Work out the finished part from the listing and answer in its coordinate system (mm). A direction names the side the tool comes from. Round coordinates to 2 decimals unless told otherwise and drop trailing zeros. Order: outer loops, then holes, each group sorted by start corner. A loop starts at its lowest first (then second) coordinate and runs counter-clockwise, first axis right, second up. Notation, with made-up numbers: (-25.5, 20.25) - (-9.5, 20.25) arc R19 cw to (-9.5, 41.25) - close; hole circle Ø10 at (-12.5, 61). An arc over 180 degrees is marked (long way). One line per question, with ' | ' between items. Start each with the question number.
Solid Edge part; units mm, degrees
sketch "Sketch1" plane through (0, 0, 0) normal (0, 0, 1) x (1, 0, 0)
  line L0 (-60, 45) -> (-60, -45)
  line L1 (-60, -45) -> (60, -45)
  line L2 (60, -45) -> (60, 45)
  line L3 (60, 45) -> (-60, 45)
extrude "Protrusion1" add sketch "Sketch1" along normal blind 15
sketch "Sketch2" plane through (0, 0, 15) normal (0, 0, 1) x (1, 0, 0)
  circle A0 centre (0, 0) radius 20
extrude "Cutout1" cut sketch "Sketch2" against normal through all
sketch "Sketch3" plane through (0, 0, 15) normal (0, 0, 1) x (1, 0, 0)
  line L0 (-60, -7.5) -> (110, -7.5)
  line L1 (110, -7.5) -> (110, 7.5)
  line L2 (110, 7.5) -> (-60, 7.5)
  line L3 (-60, 7.5) -> (-60, -7.5)
  dimension "D1" = 60
  dimension "D2" = 60
extrude "VaciadoExtruido_2" cut sketch "Sketch3" against normal blind 5
chamfer "Chaflán_1" distance 5 angle 45 4 edges at (-60, 45, 7.5) (60, 45, 7.5) (60, -45, 7.5) (-60, -45, 7.5)
hole "Agujero_1" [suppressed]
hole "Hole1" at (-35, 0, 0) direction (0, 0, 1) diameter 7 end up to next counterbore diameter 11 counterbore depth 6.8
hole "Hole2" at (50, 0, 0) direction (0, 0, 1) diameter 7 end up to next counterbore diameter 11 counterbore depth 6.8
hole "Agujero_4" at (-43, 38, 15) direction (0, 0, -1) diameter 7 end up to next counterbore diameter 11 counterbore depth 6.8
hole "Hole3" at (43, 38, 15) direction (0, 0, -1) diameter 7 end up to next counterbore diameter 11 counterbore depth 6.8
hole "Hole4" at (43, -38, 15) direction (0, 0, -1) diameter 7 end up to next counterbore diameter 11 counterbore depth 6.8
hole "Hole5" at (-43, -38, 15) direction (0, 0, -1) diameter 7 end up to next counterbore diameter 11 counterbore depth 6.8
hole "Agujero_8" at (0, 38, 15) direction (0, 0, -1) diameter 8 end up to next
hole "Hole6" at (0, -38, 15) direction (0, 0, -1) diameter 8 end up to next
properties part number "1976-1200-002" material "Aluminio, 7075-T6"
1) Section C-C on x = 43 is taken. Give the vertices of the cut face in (y, z), and give its area (3 significant figures).
2) A flat-ended cylindrical pin translates along its axis: pin 1 (5.5 mm diameter, centred on x = 42.5, y = 36, fed in from +Z). Find the tip coordinate at first contact, or state that the pin passes through.
3) For faces 1 (the flat face through (-43, -42, 8.2)), 2 (the cylindrical face through (44.547, -0.716, 3.448)), 3 (the flat face through (-1, 27, 15)), 4 (the flat face through (-40, -7.5, 13)), 5 (the cylindrical face through (46.47, 38.46, 4.16)), determine the directions among +Z, -Z, +X, -X, +Y, -Y from which every point of the face is accessible in a straight line to the end or side of a thin tool.
4) Section D-D on y = 38 is taken. Give the vertices of the cut face in (x, z).
5) Determine the mould class of faces 6 (the flat face through (58, -42, 8)), 7 (the flat face through (-60, 1, 7)), 8 (the cylindrical face through (46.47, -37.54, 4.16)) for opening direction X: released by +X, released by -X, zero draft, split by the parting line, or undercut.
6) Straight lines are drawn through the part: line 1 (X direction, y = 38, z = 12.5); line 2 (Y direction, x = -43, z = 4.75); line 3 (X direction, y = -38, z = 2.25). For each, find the intervals that lie inside material, in ascending order.
7) Section A-A on z = 11.75 is taken. Give the vertices of the cut face in (x, y).
8) Section B-B on y = -12 is taken. Give the vertices of the cut face in (x, z), and give its area (3 significant figures).
Recorded:
1) outline: (-45, 0) - (-41.5, 0) - (-41.5, 8.2) - (-43.5, 8.2) - (-43.5, 15) - (-45, 15) - close; (-34.5, 0) - (34.5, 0) - (34.5, 8.2) - (32.5, 8.2) - (32.5, 15) - (7.5, 15) - (7.5, 10) - (-7.5, 10) - (-7.5, 15) - (-32.5, 15) - (-32.5, 8.2) - (-34.5, 8.2) - close; (41.5, 0) - (45, 0) - (45, 15) - (43.5, 15) - (43.5, 8.2) - (41.5, 8.2) - close | area: 1,010 mm²
2) pin 1: stops at z = 8.2
3) face 1: +Z | face 2: -Z | face 3: +Z, +X, -X, +Y, -Y | face 4: +Z, +X, -X | face 5: +Z, -Z
4) outline: (-60, 0) - (-46.5, 0) - (-46.5, 8.2) - (-48.5, 8.2) - (-48.5, 15) - (-60, 15) - close; (-39.5, 0) - (-4, 0) - (-4, 15) - (-37.5, 15) - (-37.5, 8.2) - (-39.5, 8.2) - close; (4, 0) - (39.5, 0) - (39.5, 8.2) - (37.5, 8.2) - (37.5, 15) - (4, 15) - close; (46.5, 0) - (60, 0) - (60, 15) - (48.5, 15) - (48.5, 8.2) - (46.5, 8.2) - close
5) face 6: released by +X | face 7: released by -X | face 8: undercut
6) line 1: x = -60 to -48.5, -37.5 to -4, 4 to 37.5, 48.5 to 60 | line 2: y = -45 to -41.5, -34.5 to 34.5, 41.5 to 45 | line 3: x = -60 to -46.5, -39.5 to -4, 4 to 39.5, 46.5 to 60
7) outline: (-60, -40) - (-55, -45) - (55, -45) - (60, -40) - (60, -7.5) - (18.54, -7.5) arc R20 cw to (-18.54, -7.5) - (-60, -7.5) - close; (-60, 7.5) - (-18.54, 7.5) arc R20 cw to (18.54, 7.5) - (60, 7.5) - (60, 40) - (55, 45) - (-55, 45) - (-60, 40) - close; hole circle Ø11 at (-43, -38); hole circle Ø11 at (-43, 38); hole circle Ø8 at (0, -38); hole circle Ø8 at (0, 38); hole circle Ø11 at (43, -38); hole circle Ø11 at (43, 38)
8) outline: (-60, 0) - (-16, 0) - (-16, 15) - (-60, 15) - close; (16, 0) - (60, 0) - (60, 15) - (16, 15) - close | area: 1,320 mm²
